For this review, take the finished solid that the model builds, in its own axes (mm). Face numbers are marked on the shaded views. A direction names the side the tool comes from. Round coordinates to 2 decimals unless told otherwise and drop trailing zeros. Order: outer loops, then holes, each group sorted by start corner. A loop starts at its lowest first (then second) coordinate and runs counter-clockwise, first axis right, second up. Notation, with made-up numbers: (4.25, 16) -> (13.25, 16) arc R6 ccw to (13.25, 23) -> close; hole circle Ø2 at (-1.75, 2). An arc over 180 degrees is marked (long way). Answer in a Markdown table with one row per item.
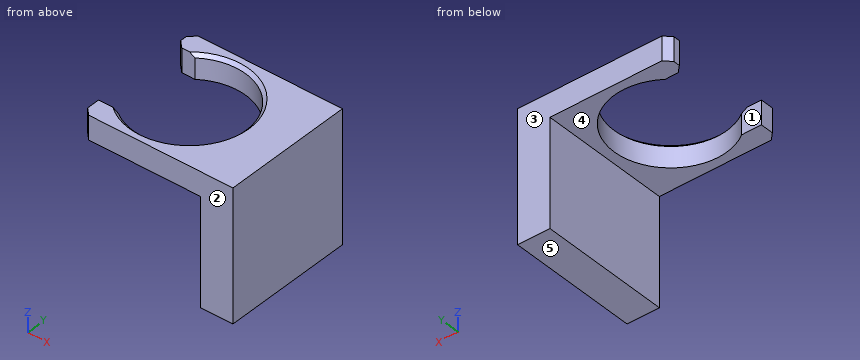
```python
from build123d import *

# Parameters (mm, degrees)
F1_DEPTH = 3.65
F2_SIZE  = 1
F3_SIZE  = 0.5
F4_W     = 4.925
F4_H     = 20
F5_DEPTH = 20


with BuildPart() as f1:
    # F0 (on Top) → F1 (new body)
    with BuildSketch(Plane.XY):
        with BuildLine():
            ThreePointArc((-4.9959983987, 7), (8.6, 0), (-4.9959983987, -7))
            Line((-4.9959983987, -7), (-8, -7))
            Line((-8, -7), (-8, -10))
            Line((-8, -10), (8, -10))
            Line((8, -10), (15, -10))
            Line((15, -10), (15, 10))
            Line((15, 10), (8, 10))
            Line((8, 10), (-8, 10))
            Line((-8, 10), (-8, 7))
            Line((-8, 7), (-4.9959983987, 7))
        make_face()
    extrude(amount=F1_DEPTH)

    # F2
    f2_edges = [f1.edges().sort_by_distance(p)[0] for p in [
        (-8, 10, 1.825),
        (-8, 7, 1.825),
        (-8, -10, 1.825),
    ]]
    chamfer(f2_edges, length=F2_SIZE)

    # F3
    f3_edges = [f1.edges().sort_by_distance(p)[0] for p in [
        (8.6, 0, 3.65),
    ]]
    chamfer(f3_edges, length=F3_SIZE)

    # F4 (on face) → F5 (join)
    with BuildSketch(Plane.XY.offset(3.65)):
        with Locations((12.5375, 0)):
            Rectangle(F4_W, F4_H)
    extrude(amount=-F5_DEPTH)


solid = f1.part
```
Q1. Take a section at A-A, the plane x = 0. Write out the cut boundary in (y, z), then the cut area to 3 significant figures.
Answer key:
| item | result |
|---|---|
| outline | (-10, 0) -> (-8.6, 0) -> (-8.6, 3.15) -> (-9.1, 3.65) -> (-10, 3.65) -> close; (8.6, 0) -> (10, 0) -> (10, 3.65) -> (9.1, 3.65) -> (8.6, 3.15) -> close |
| area | 9.97 mm^2 |
Q2. Clearance check with flat-ended pins moving along their axes: pin 1 Ø12 at (x, y) = (-3.5, -2.5) entering from -Z; pin 2 Ø5 at (y, z) = (2, -7.5) entering from -X (3 decimals); pin 3 Ø5 at (x, z) = (9.5, -2) entering from -Y. State where each tip first meets the part, or that it passes through.
Answer key:
| item | result |
|---|---|
| pin 1 | stops at z = 0 |
| pin 2 | stops at x = 10.075 |
| pin 3 | stops at y = -10 |
Q3. Take a section at B-B, the plane z = 0.75. Write out the cut boundary in (x, y), then the cut area to 3 significant figures.
Answer key:
| item | result |
|---|---|
| outline | (-8, -9) -> (-7, -10) -> (15, -10) -> (15, 10) -> (-7, 10) -> (-8, 9) -> (-8, 8) -> (-7, 7) -> (-5, 7) arc R8.6 cw (long way) to (-5, -7) -> (-8, -7) -> close |
| area | 219 mm^2 |
Q4. Tool access review of the marked faces 4 and 5: name each direction out of +Z, -Z, +X, -X, +Y, -Y from which nothing blocks a thin tool from reaching the whole face with its end or side.
Answer key:
| item | result |
|---|---|
| face 4 | -Z, -X, +Y, -Y |
| face 5 | -Z, +X, -X, +Y, -Y |
Q5. Take a section at D-D, the plane z = -9.25. Write out the cut boundary in (x, y) (3 decimals).
Answer key:
| item | result |
|---|---|
| outline | (10.075, -10) -> (15, -10) -> (15, 10) -> (10.075, 10) -> close |
Q6. The part is to be moulded in two halves that separate along Y. For the marked faces 1, 2 and 3, say which applies: +Y half, -Y half, draft (parallel to the pull), parting line (faces both ways), or undercut.
Answer key:
| item | result |
|---|---|
| face 1 | undercut |
| face 2 | -Y half |
| face 3 | +Y half |
Q7. To check wall thickness, follow probe 1 along Y at (x, z) = (0, 2.4); probe 2 along X at (y, z) = (-5.75, -7.25) (3 decimals); probe 3 along Z at (x, y) = (7.5, -6). State the ranges of each line that lie inside material, in increasing order.
Answer key:
| item | result |
|---|---|
| probe 1 | y = -10 to -8.6, 8.6 to 10 |
| probe 2 | x = 10.075 to 15 |
| probe 3 | z = 0 to 3.65 |
Q8. Take a section at C-C, the plane y = 0. Write out the cut boundary in (x, z) (3 decimals).
Answer key:
| item | result |
|---|---|
| outline | (8.6, 0) -> (10.075, 0) -> (10.075, -16.35) -> (15, -16.35) -> (15, 3.65) -> (9.1, 3.65) -> (8.6, 3.15) -> close |
